```python
from build123d import *

# Parameters (mm, degrees)
SKETCH_1_W          = 160
SKETCH_1_H          = 160
EXTRUDE_1_DEPTH     = 2
SKETCH_2_W          = 70
SKETCH_2_H          = 65
EXTRUDE_2_DEPTH     = 2
SKETCH_3_R          = 2.1
CUT_EXTRUDE_1_DEPTH = 166.61702811
SKETCH_4_R          = 15
CUT_EXTRUDE_2_DEPTH = 10
FILLET_1_R          = 2
SKETCH_5_R          = 1.6
CUT_EXTRUDE_3_DEPTH = 10


with BuildPart() as part:
    # 草图1 → 凸台-拉伸1 (new body)
    with BuildSketch(Plane.XY):
        Rectangle(SKETCH_1_W, SKETCH_1_H)
    extrude(amount=EXTRUDE_1_DEPTH)

    # 草图2 → 凸台-拉伸2 (add, through all)
    with BuildSketch(Plane.XY.offset(2)):
        with Locations((-20, -112.5)):
            Rectangle(SKETCH_2_W, SKETCH_2_H)
    extrude(amount=-EXTRUDE_2_DEPTH)

    # 草图3 → 切除-拉伸1 (cut, through all)
    with BuildSketch(Plane.XY.offset(2)):
        with Locations((-70, 70)):
            Circle(SKETCH_3_R)
        with Locations((-50, 70)):
            Circle(SKETCH_3_R)
        with Locations((-70, 50)):
            Circle(SKETCH_3_R)
    extrude(amount=-CUT_EXTRUDE_1_DEPTH, mode=Mode.SUBTRACT)

    # 草图4 → 切除-拉伸2 (cut)
    with BuildSketch(Plane.XY.offset(2)):
        with Locations((-20, -112.5)):
            Circle(SKETCH_4_R)
        with BuildLine():
            Line((-25, 72.1), (75, 72.1))
            ThreePointArc((75, 72.1), (77.1, 70), (75, 67.9))
            Line((75, 67.9), (-25, 67.9))
            ThreePointArc((-25, 67.9), (-27.1, 70), (-25, 72.1))
        make_face()
        with BuildLine():
            Line((-67.9, 30), (-67.9, -70))
            ThreePointArc((-67.9, -70), (-70, -72.1), (-72.1, -70))
            Line((-72.1, -70), (-72.1, 30))
            ThreePointArc((-72.1, 30), (-70, 32.1), (-67.9, 30))
        make_face()
        with BuildLine():
            Line((-25, 56.1), (75, 56.1))
            ThreePointArc((75, 56.1), (77.1, 54), (75, 51.9))
            Line((75, 51.9), (-25, 51.9))
            ThreePointArc((-25, 51.9), (-27.1, 54), (-25, 56.1))
        make_face()
        with BuildLine():
            Line((-25, 40.1), (75, 40.1))
            ThreePointArc((75, 40.1), (77.1, 38), (75, 35.9))
            Line((75, 35.9), (-25, 35.9))
            ThreePointArc((-25, 35.9), (-27.1, 38), (-25, 40.1))
        make_face()
        with BuildLine():
            Line((-25, 24.1), (75, 24.1))
            ThreePointArc((75, 24.1), (77.1, 22), (75, 19.9))
            Line((75, 19.9), (-25, 19.9))
            ThreePointArc((-25, 19.9), (-27.1, 22), (-25, 24.1))
        make_face()
        with BuildLine():
            Line((-25, 8.1), (75, 8.1))
            ThreePointArc((75, 8.1), (77.1, 6), (75, 3.9))
            Line((75, 3.9), (-25, 3.9))
            ThreePointArc((-25, 3.9), (-27.1, 6), (-25, 8.1))
        make_face()
        with BuildLine():
            Line((-25, -7.9), (75, -7.9))
            ThreePointArc((75, -7.9), (77.1, -10), (75, -12.1))
            Line((75, -12.1), (-25, -12.1))
            ThreePointArc((-25, -12.1), (-27.1, -10), (-25, -7.9))
        make_face()
        with BuildLine():
            Line((-25, -23.9), (75, -23.9))
            ThreePointArc((75, -23.9), (77.1, -26), (75, -28.1))
            Line((75, -28.1), (-25, -28.1))
            ThreePointArc((-25, -28.1), (-27.1, -26), (-25, -23.9))
        make_face()
        with BuildLine():
            Line((-25, -39.9), (75, -39.9))
            ThreePointArc((75, -39.9), (77.1, -42), (75, -44.1))
            Line((75, -44.1), (-25, -44.1))
            ThreePointArc((-25, -44.1), (-27.1, -42), (-25, -39.9))
        make_face()
        with BuildLine():
            Line((-25, -55.9), (75, -55.9))
            ThreePointArc((75, -55.9), (77.1, -58), (75, -60.1))
            Line((75, -60.1), (-25, -60.1))
            ThreePointArc((-25, -60.1), (-27.1, -58), (-25, -55.9))
        make_face()
        with BuildLine():
            Line((-25, -71.9), (75, -71.9))
            ThreePointArc((75, -71.9), (77.1, -74), (75, -76.1))
            Line((75, -76.1), (-25, -76.1))
            ThreePointArc((-25, -76.1), (-27.1, -74), (-25, -71.9))
        make_face()
        with BuildLine():
            Line((-57.1, 30), (-57.1, -70))
            ThreePointArc((-57.1, -70), (-55, -72.1), (-52.9, -70))
            Line((-52.9, -70), (-52.9, 30))
            ThreePointArc((-52.9, 30), (-55, 32.1), (-57.1, 30))
        make_face()
        with BuildLine():
            Line((-42.1, 30), (-42.1, -70))
            ThreePointArc((-42.1, -70), (-40, -72.1), (-37.9, -70))
            Line((-37.9, -70), (-37.9, 30))
            ThreePointArc((-37.9, 30), (-40, 32.1), (-42.1, 30))
        make_face()
    extrude(amount=-CUT_EXTRUDE_2_DEPTH, mode=Mode.SUBTRACT)

    # 圆角1
    fillet_1_edges = [part.edges().sort_by_distance(p)[0] for p in [
        (15, -145, 1),
        (-55, -145, 1),
        (80, -80, 1),
        (-80, -80, 1),
        (-80, 80, 1),
        (80, 80, 1),
    ]]
    fillet(fillet_1_edges, radius=FILLET_1_R)

    # 草图5 → 切除-拉伸3 (cut)
    with BuildSketch(Plane.XY.offset(2)):
        with Locations((35, 30.9)):
            Circle(SKETCH_5_R)
        with Locations((3, 30.9)):
            Circle(SKETCH_5_R)
        with Locations((3, -34.1)):
            Circle(SKETCH_5_R)
        with Locations((35, -34.1)):
            Circle(SKETCH_5_R)
    extrude(amount=-CUT_EXTRUDE_3_DEPTH, mode=Mode.SUBTRACT)


solid = part.part
```
Model file for the job. Use its own axes, mm. Give positions to 0.01 mm unless a question says otherwise; leave off trailing zeros. Loops run counter-clockwise (first coordinate to the right, second up) from the corner with the lowest first, then second, coordinate; pieces in that order, holes last. Notation, with made-up numbers: (75.5, -11.75) - (87.5, -11.75) arc R26 cw to (87.5, 2.25) - close; hole circle Ø1 at (-26, 18.5). An arc over 180 degrees is marked (long way). One line per item, written item: value. Start each with the question number.
1. Slice it at C-C (x = 26.5). Give the number of separate pieces and of enclosed holes in the cut face, plus the area to 3 significant figures.
2. Pin check, flat tips, straight feed: pin 1 (3 mm diameter, centred on x = 35, y = 30.9, fed in from -Z); pin 2 (0.6 mm diameter, centred on x = 34.5, z = 1.5, fed in from -Y); pin 3 (5.5 mm diameter, centred on x = -70, y = 70, fed in from -Z). Stop position of each tip, or through.
3. Pull direction X, two halves, no side cores. Call faces 1 (the cylindrical face through (-48.06, 69.2, 1.01)), 2 (the flat face through (-1, -6, 0)): pulls with the +X half, pulls with the -X half, needs draft (parallel to the pull), parting line crosses it, or undercut.
4. Probe L1, parallel to X at y = 10, z = 1.6; L2, parallel to X at y = -35.5, z = 1.7; L3, parallel to X at y = 31, z = 1.8. List the from-to ranges inside material, lowest first. Write a range as from..to.
5. Slice it at A-A (y = 13.5). List the corners of the cut face in (x, z), plus the area to 3 significant figures.
6. Slice it at B-B (x = -32). List the corners of the cut face in (y, z), plus the area to 3 significant figures.
Solution:
1. separate pieces: 11
1. enclosed holes: 0
1. area: 236 mm^2
2. pin 1: passes through
2. pin 2: stops at y = -80
2. pin 3: stops at z = 0
3. face 1: undercut
3. face 2: needs draft
4. L1: x = -80..-72.1, -67.9..-57.1, -52.9..-42.1, -37.9..80
4. L2: x = -80..-72.1, -67.9..-57.1, -52.9..-42.1, -37.9..2.23, 3.77..34.23, 35.77..80
4. L3: x = -80..-71.85, -68.15..-56.85, -53.15..-41.85, -38.15..1.4, 4.6..33.4, 36.6..80
5. outline: (-80, 0) - (-72.1, 0) - (-72.1, 2) - (-80, 2) - close; (-67.9, 0) - (-57.1, 0) - (-57.1, 2) - (-67.9, 2) - close; (-52.9, 0) - (-42.1, 0) - (-42.1, 2) - (-52.9, 2) - close; (-37.9, 0) - (80, 0) - (80, 2) - (-37.9, 2) - close
5. area: 295 mm^2
6. outline: (-145, 0) - (-121.5, 0) - (-121.5, 2) - (-145, 2) - close; (-103.5, 0) - (80, 0) - (80, 2) - (-103.5, 2) - close
6. area: 414 mm^2
